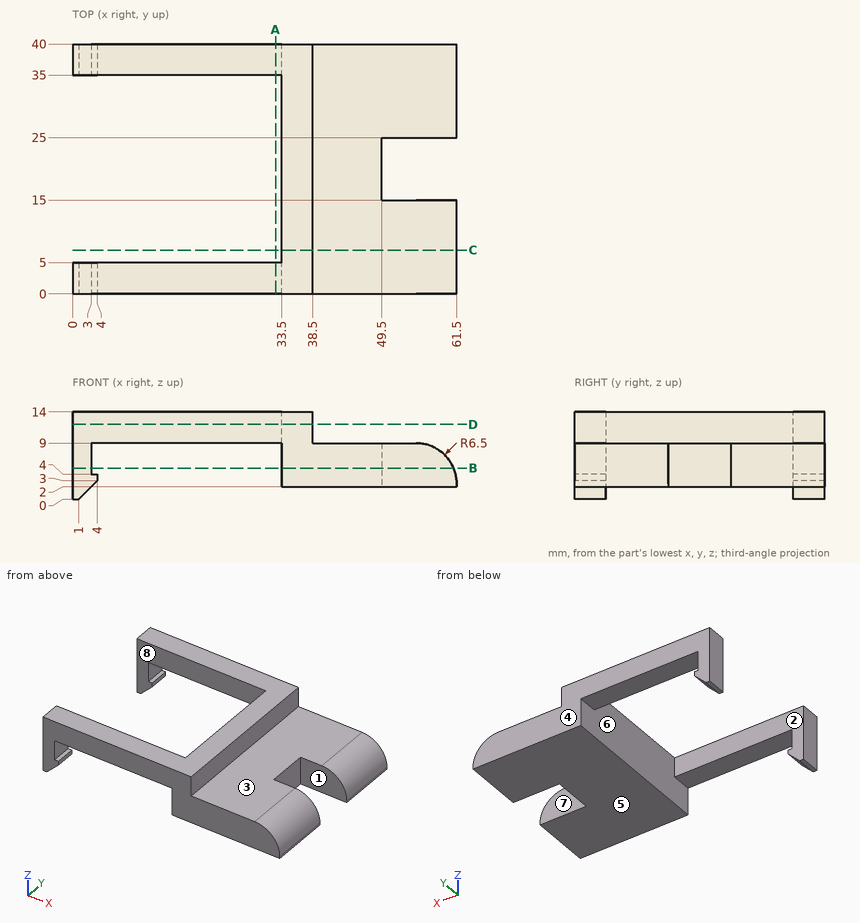
Verification items for this drawing (mm, ordinates from the low corner). A direction names the side the tool comes from. Coordinates: 2 decimals unless noted, no trailing zeros. Write each loop counter-clockwise with the first axis right and the second up, starting at its lowest first coordinate (ties: lowest second). Pieces come first, ordered by that corner, then holes. Notation, with made-up numbers: M 81.5,54.5 L 96.5,54.5 A26 ccw 96.5,93.5 Z; hole C 8,85 d3. An arc over 180 degrees is marked long. Answer as a JSON object with one key per item and string values.
1. Section check D-D, the plane z = 12. Enter the section's corners in (x, y).
Answers below:
{"outline": "M 0,0 L 38.5,0 L 38.5,40 L 0,40 L 0,35 L 33.5,35 L 33.5,5 L 0,5 Z"}
2. Section check A-A, the plane x = 32.5. Enter the section's corners in (y, z).
Answers below:
{"outline": "M 0,9 L 5,9 L 5,14 L 0,14 Z; M 35,9 L 40,9 L 40,14 L 35,14 Z"}
3. Go/stop test with flat-tipped pins: pin 1 Ø3 at (y, z) = (33.5, 7) entering from +X; pin 2 Ø2 at (y, z) = (20, 4.5) entering from +X; pin 3 Ø0.5 at (y, z) = (2, 3.5) entering from +X; pin 4 Ø6 at (x, z) = (24, 4.5) entering from +Y. Record where each tip stops, or that it passes through.
Answers below:
{"pin 1": "stops at x = 60.77", "pin 2": "stops at x = 49.5", "pin 3": "stops at x = 61.46", "pin 4": "passes through"}
4. Draft check along Y on the marked faces 1, 2, 3 and 4. Enter one of: released by +Y, released by -Y, zero draft, split by the parting line, or undercut.
Answers below:
{"face 1": "undercut", "face 2": "undercut", "face 3": "zero draft", "face 4": "released by +Y"}
5. Section check C-C, the plane y = 7. Enter the section's corners in (x, z).
Answers below:
{"outline": "M 33.5,2 L 61.5,2 L 61.5,2.5 A6.5 ccw 55,9 L 38.5,9 L 38.5,14 L 33.5,14 Z"}
6. Tool access check on the marked faces 5, 6, 7 and 8. Record the directions out of +Z, -Z, +X, -X, +Y, -Y that give a thin tool (end or side, any length) a straight path to the whole face; none if there is none.
Answers below:
{"face 5": "-Z, +X, +Y, -Y", "face 6": "-Z", "face 7": "+Z, -Z, +X", "face 8": "+Z, -Z, -X"}
7. Section check B-B, the plane z = 5. Enter the section's corners in (x, y), plus the area to 4 significant figures.
Answers below:
{"outline": "M 0,0 L 3,0 L 3,5 L 0,5 Z; M 0,35 L 3,35 L 3,40 L 0,40 Z; M 33.5,0 L 61,0 L 61,15 L 49.5,15 L 49.5,25 L 61,25 L 61,40 L 33.5,40 Z", "area": "1,015 mm²"}
8. Scan lines: L1, parallel to Y at x = 23.5, z = 11.5; L2, parallel to Y at x = 57, z = 8; L3, parallel to Z at x = 14.5, y = 2. Record each from-to range of solid material in increasing order.
Answers below:
{"L1": "y = 0 to 5, 35 to 40", "L2": "y = 0 to 15, 25 to 40", "L3": "z = 9 to 14"}
